from build123d import *
from OCP.BRepFilletAPI import BRepFilletAPI_MakeChamfer

# Parameters (mm, degrees)
SKICA1_R                 = 4
P_IDAT_VYSUNUT_M1_DEPTH  = 148
ZKOSEN_1_SIZE            = 0.5
ZKOSEN_1_SIZE2           = 0.233153829
ODEBRAT_START            = -20
ODEBRAT_VYSUNUT_M1_DEPTH = 20


with BuildPart() as part:
    # Skica1 → Přidat vysunutím1 (new body)
    with BuildSketch(Plane.XY):
        Circle(SKICA1_R)
    extrude(amount=P_IDAT_VYSUNUT_M1_DEPTH)

    # Zkosení1: one chamfer whose edges measure the first distance from different faces: ONE call of the kernel's chamfer builder (chamfer() names one face for all edges)
    zkosen_1_edges_1 = [part.edges().sort_by_distance(p)[0] for p in [
        (-4, 0, 0),
    ]]
    zkosen_1_side_1 = [part.faces().sort_by_distance(p)[0] for p in [
        (0, 0, 0),
    ]]
    zkosen_1_edges_2 = [part.edges().sort_by_distance(p)[0] for p in [
        (-4, 0, 148),
    ]]
    zkosen_1_side_2 = [part.faces().sort_by_distance(p)[0] for p in [
        (-4, 0, 74),
    ]]
    zkosen_1 = BRepFilletAPI_MakeChamfer(part.part.solid().wrapped)
    for e in zkosen_1_edges_1:
        zkosen_1.Add(ZKOSEN_1_SIZE, ZKOSEN_1_SIZE2, e.wrapped, zkosen_1_side_1[0].wrapped)  # the first distance lies on this face
    for e in zkosen_1_edges_2:
        zkosen_1.Add(ZKOSEN_1_SIZE, ZKOSEN_1_SIZE2, e.wrapped, zkosen_1_side_2[0].wrapped)  # the first distance lies on this face
    add(Compound.cast(zkosen_1.Shape()), mode=Mode.REPLACE)

    # Skica2 → Odebrat vysunutím1 (cut)
    with BuildSketch(Plane.XY.offset(148).offset(ODEBRAT_START)):
        with BuildLine():
            Line((-1.936491673, 3.5), (1.936491673, 3.5))
            ThreePointArc((1.936491673, 3.5), (0, 4), (-1.936491673, 3.5))
        make_face()
    extrude(amount=ODEBRAT_VYSUNUT_M1_DEPTH, mode=Mode.SUBTRACT)


solid = part.part
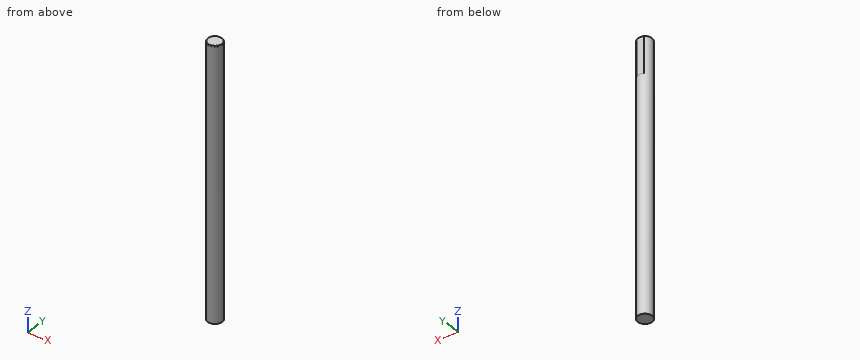
Here's how the part is built. I have some questions about the finished solid (model axes, mm). Round coordinates to 2 decimals unless told otherwise and drop trailing zeros. Loops run counter-clockwise (first coordinate to the right, second up) from the corner with the lowest first, then second, coordinate; pieces in that order, holes last.
1. For P1, Ø3, axis at x = 1, z = 139.5, coming from the +Y side, with a flat end and sliding along its axis, tell me the tip position at first contact or that it passes through.
Answer list:
P1: stops at y = 3.5
2. If we section it at A-A on z = 83: Write out the boundary of the cut face in (x, y), plus the area to 3 significant figures.
Answer list:
outline: circle Ø8 at (0, 0)
area: 50.3 mm2
3. If I drill on line 1 along X through (y, z) = (3.5, 70); line 2 along Y through (x, z) = (0.25, 46); line 3 along X through (y, z) = (3.25, 27), over which ranges is the centre line in solid material (lowest first)?
Answer list:
line 1: x = -1.94 to 1.94
line 2: y = -3.99 to 3.99
line 3: x = -2.33 to 2.33
